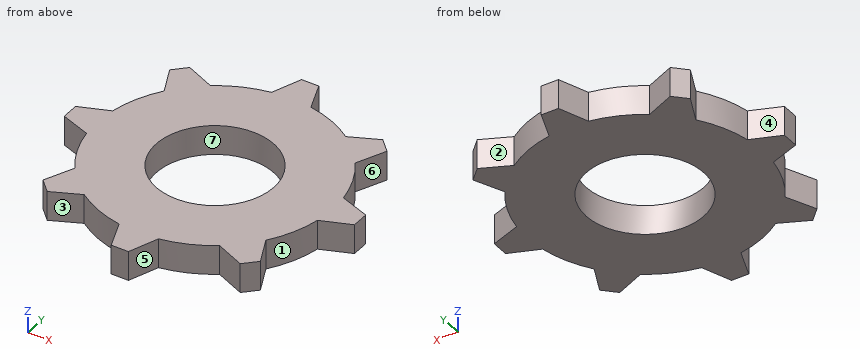
from build123d import *

# Parameters (mm, degrees)
CROQUIS1_R              = 8
CROQUIS1_R_2            = 4
SALIENTE_EXTRUIR5_DEPTH = 2
SALIENTE_EXTRUIR7_DEPTH = 2
MATRIZC5_COUNT          = 8


with BuildPart() as part:
    # Croquis1 → Saliente-Extruir5 (new body)
    with BuildSketch(Plane.XY):
        Circle(CROQUIS1_R)
        Circle(CROQUIS1_R_2, mode=Mode.SUBTRACT)
    extrude(amount=SALIENTE_EXTRUIR5_DEPTH)

    # Croquis5 → Saliente-Extruir7 (add)
    with BuildSketch(Plane.XY):
        Polygon((0.009306697, 9.894487771), (-0.577837412, 9.894487771), (-1.314748981, 7.891225198), (-1.314748981, 7.565133639), (1.376804344, 7.565133639), (1.376804344, 7.880635114), (0.594453217, 9.894487771), align=None)
    saliente_extruir7 = extrude(amount=SALIENTE_EXTRUIR7_DEPTH)

    # MatrizC5: Saliente-Extruir7 ×8 about axis
    matrizc5_axis = Axis((0, 0, 0), (0, 0, 1))
    for i in range(1, MATRIZC5_COUNT):
        add(saliente_extruir7.rotate(matrizc5_axis, i * 360 / MATRIZC5_COUNT))


solid = part.part
Design review of the part built by this model. Coordinates are the model's own, in mm. Face numbers are marked on the shaded views. A direction names the side the tool comes from. Round coordinates to 2 decimals unless told otherwise and drop trailing zeros. Loops run counter-clockwise (first coordinate to the right, second up) from the corner with the lowest first, then second, coordinate; pieces in that order, holes last. Notation, with made-up numbers: (-25.75, 39) -> (7.25, 39) arc R26 ccw to (7.25, 71) -> close; hole circle Ø10 at (71, 65.5). An arc over 180 degrees is marked (long way). Use one line per item in the form item = value. Start each with the question number.
Q1. For pin 1 Ø3 at (x, y) = (-7, -7.5) entering from +Z, flat-tipped, find the tip position at first contact; note if it passes through.
Q2. Wall thickness on line 1 along Y through (x, z) = (0, 1.6); line 2 along Y through (x, z) = (6.75, 1.8); line 3 along X through (y, z) = (-7, 1.8): over which ranges is each line inside the solid? List them lowest first. Write a range as [from, to].
Q3. We need section A-A on y = 0. Give the boundary of the cut face in (x, z).
Q4. Machinability: for the marked faces 1, 2 and 3, which of the approach directions +Z, -Z, +X, -X, +Y, -Y give a long, thin tool a straight path to every point of the face, cutting with its end or side? Answer none if there is none.
Q5. Draft analysis for pull direction Y (two halves, no side actions). For the marked faces 4, 5, 6 and 7, state which applies: +Y half, -Y half, draft (parallel to the pull), parting line (faces both ways), or undercut.
Q6. We need section D-D on x = 8.25. Give the boundary of the cut face in (y, z).
Calculated:
q1.pin_1 = 2
q2.line_1 = [-9.89, -4], [4, 9.89]
q2.line_2 = [-7.24, -5.17], [-4.29, 4.29], [5.06, 7.24]
q2.line_3 = [-6.99, -5.71], [-3.87, 3.87], [5.63, 6.99]
q3.outline = (-9.89, 0) -> (-4, 0) -> (-4, 2) -> (-9.89, 2) -> close; (4, 0) -> (9.89, 0) -> (9.89, 2) -> (4, 2) -> close
q4.face_1 = +Z, -Z, +X
q4.face_2 = +Z, -Z, +Y
q4.face_3 = +Z, -Z, -Y
q5.face_4 = +Y half
q5.face_5 = -Y half
q5.face_6 = undercut
q5.face_7 = undercut
q6.outline = (-1.23, 0) -> (1.18, 0) -> (1.18, 2) -> (-1.23, 2) -> close
